```python
from build123d import *

# Parameters (mm, degrees)
SKETCH_1_R      = 1.5
SKETCH_1_W      = 9.7
SKETCH_1_H      = 1.95
SKETCH_1_W_2    = 5
EXTRUDE_1_DEPTH = 3


with BuildPart() as part:
    # Эскиз1 → Бобышка-Вытянуть1 (new body)
    with BuildSketch(Plane.XY):
        with BuildLine():
            Line((-69.489291724, -55), (69.489291724, -55))
            ThreePointArc((69.489291724, -55), (74.489291724, -53.660254038), (78.149545762, -50))
            Line((78.149545762, -50), (82.37604307, -42.679491924))
            ThreePointArc((82.37604307, -42.679491924), (83.715789032, -37.679491924), (82.37604307, -32.679491924))
            Line((82.37604307, -32.679491924), (12.886751346, 87.679491924))
            ThreePointArc((12.886751346, 87.679491924), (9.226497308, 91.339745962), (4.226497308, 92.679491924))
            Line((4.226497308, 92.679491924), (-4.226497308, 92.679491924))
            ThreePointArc((-4.226497308, 92.679491924), (-9.226497308, 91.339745962), (-12.886751346, 87.679491924))
            Line((-12.886751346, 87.679491924), (-82.37604307, -32.679491924))
            ThreePointArc((-82.37604307, -32.679491924), (-83.715789032, -37.679491924), (-82.37604307, -42.679491924))
            Line((-82.37604307, -42.679491924), (-78.149545762, -50))
            ThreePointArc((-78.149545762, -50), (-74.489291724, -53.660254038), (-69.489291724, -55))
        make_face()
        with Locations((-76.798692801, -44.339745962)):
            Circle(SKETCH_1_R, mode=Mode.SUBTRACT)
        with Locations(Location((0, 88.679491924, 0), (0, 0, 180))):
            Circle(SKETCH_1_R, mode=Mode.SUBTRACT)
        with Locations((76.798692801, -44.339745962)):
            Circle(SKETCH_1_R, mode=Mode.SUBTRACT)
        Polygon((-71.342603888, -46.789969171), (-76.192603888, -38.389522754), (-74.503854351, -37.414522754), (-69.653854351, -45.814969171), align=None, mode=Mode.SUBTRACT)
        with Locations((0, 84.204491924)):
            Rectangle(SKETCH_1_W, SKETCH_1_H, mode=Mode.SUBTRACT)
        Polygon((76.192603888, -38.389522754), (71.342603888, -46.789969171), (69.653854351, -45.814969171), (74.503854351, -37.414522754), align=None, mode=Mode.SUBTRACT)
        Polygon((-64.84741336, -43.039969171), (-69.69741336, -34.639522754), (-68.008663822, -33.664522754), (-63.158663822, -42.064969171), align=None, mode=Mode.SUBTRACT)
        with Locations((0, 76.704491924)):
            Rectangle(SKETCH_1_W, SKETCH_1_H, mode=Mode.SUBTRACT)
        Polygon((69.69741336, -34.639522754), (64.84741336, -43.039969171), (63.158663822, -42.064969171), (68.008663822, -33.664522754), align=None, mode=Mode.SUBTRACT)
        Polygon((70.508663822, -29.334395735), (72.19741336, -30.309395735), (74.69741336, -25.979268716), (73.008663822, -25.004268716), align=None, mode=Mode.SUBTRACT)
        Polygon((62.34741336, -47.370096189), (59.84741336, -51.700223208), (58.158663822, -50.725223208), (60.658663822, -46.395096189), align=None, mode=Mode.SUBTRACT)
        with Locations((-12.35, 76.704491924)):
            Rectangle(SKETCH_1_W_2, SKETCH_1_H, mode=Mode.SUBTRACT)
        with Locations((12.35, 76.704491924)):
            Rectangle(SKETCH_1_W_2, SKETCH_1_H, mode=Mode.SUBTRACT)
        Polygon((-60.658663822, -46.395096189), (-62.34741336, -47.370096189), (-59.84741336, -51.700223208), (-58.158663822, -50.725223208), align=None, mode=Mode.SUBTRACT)
        Polygon((-70.508663822, -29.334395735), (-73.008663822, -25.004268716), (-74.69741336, -25.979268716), (-72.19741336, -30.309395735), align=None, mode=Mode.SUBTRACT)
    extrude(amount=EXTRUDE_1_DEPTH)


solid = part.part
```
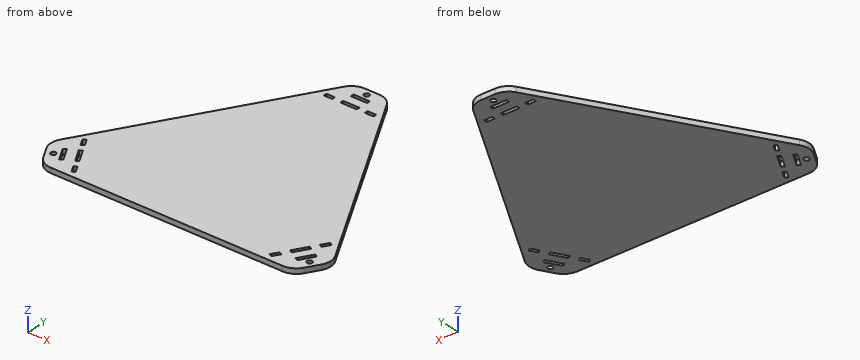
Model file for the job. Use its own axes, mm. Coordinates: 2 decimals unless noted, no trailing zeros. Write each loop counter-clockwise with the first axis right and the second up, starting at its lowest first coordinate (ties: lowest second). Pieces come first, ordered by that corner, then holes. Notation, with made-up numbers: (-31.75, 11) - (20.25, 11) arc R24 ccw to (20.25, 44) - close; hole circle Ø9 at (-19.75, 17.5). An arc over 180 degrees is marked (long way). One line per item, written item: value. Start each with the question number.
1. Probe line 1 (X direction, y = -30, z = 2.05); line 2 (X direction, y = -13.5, z = 2.45); line 3 (X direction, y = 77.5, z = 0.6). List the from-to ranges inside material, lowest first. Write a range as from..to.
2. Slice it at A-A (z = 2.05). Count the separate pieces of the cut face and the enclosed holes in it, plus the area to 3 significant figures.
3. Slice it at C-C (y = 69). Write the cut outline in (x, z), plus the area to 3 significant figures.
4. Flat gauge pins, fed straight in: pin 1 (1.8 mm diameter, centred on x = 76.8, y = -44.34, fed in from -Z); pin 2 (1 mm diameter, centred on x = -34.5, z = 0.5, fed in from +Y); pin 3 (0.6 mm diameter, centred on y = 77, z = 1, fed in from +X); pin 4 (0.6 mm diameter, centred on y = 77, z = 2, fed in from -X). Where does each tip first touch, or does it go through?
5. Slice it at B-B (x = -24). Write the cut outline in (y, z).
Answers below:
1. line 1: x = -80.83..-72.38, -71.66..71.66, 72.38..80.83
1. line 2: x = -71.3..71.3
1. line 3: x = -18.76..-14.85, -9.85..-4.85, 4.85..9.85, 14.85..18.76
2. separate pieces: 1
2. enclosed holes: 15
2. area: 15,000 mm^2
3. outline: (-23.67, 0) - (23.67, 0) - (23.67, 3) - (-23.67, 3) - close
3. area: 142 mm^2
4. pin 1: passes through
4. pin 2: stops at y = 51.11
4. pin 3: stops at x = 19.23
4. pin 4: stops at x = -19.23
5. outline: (-55, 0) - (68.43, 0) - (68.43, 3) - (-55, 3) - close
